The model under review builds one solid part; all positions refer to its coordinate system, in mm. Coordinates: 2 decimals unless noted, no trailing zeros. Order: outer loops, then holes, each group sorted by start corner. A loop starts at its lowest first (then second) coordinate and runs counter-clockwise, first axis right, second up.
from build123d import *

# Parameters (mm, degrees)
SKETCH1_W          = 127
SKETCH1_H          = 190.5
BASE_FLANGE1_DEPTH = 3.175
SKETCH7_R          = 2.54
SKETCH7_R_2        = 3.175
SKETCH7_R_3        = 14.2875
CUT_EXTRUDE1_DEPTH = 3.175
SKETCH10_R         = 2.54
CUT_EXTRUDE2_DEPTH = 115.52027386
CUT_EXTRUDE3_DEPTH = 115.52027386
CUT_EXTRUDE4_DEPTH = 115.52027386
SKETCH13_R         = 2.54
CUT_EXTRUDE5_DEPTH = 115.52027386


# Sheet-metal steps are written as plain solids
with BuildPart() as part:
    # Sketch1 → Base-Flange1 (new body)
    with BuildSketch(Plane(origin=(0, 0, 0), x_dir=(0, 0, -1), z_dir=(1, 0, 0))):
        Rectangle(SKETCH1_W, SKETCH1_H)
    extrude(amount=-BASE_FLANGE1_DEPTH)

    # Sketch7 → Cut-Extrude1 (cut)
    with BuildSketch(Plane(origin=(0, 0, 0), x_dir=(0, 0, -1), z_dir=(1, 0, 0))):
        with Locations((-28.380000009, -53.975)):
            Circle(SKETCH7_R)
        with Locations((28.380000009, -53.975)):
            Circle(SKETCH7_R)
        with Locations((0, 43.476657776)):
            Circle(SKETCH7_R_2)
        with Locations((0, -5.249171112)):
            Circle(SKETCH7_R_3)
    extrude(amount=-CUT_EXTRUDE1_DEPTH, mode=Mode.SUBTRACT)

    # Sketch10 → Cut-Extrude2 (cut, through all)
    with BuildSketch(Plane.ZY.offset(3.175)):
        with Locations((0, 34.740957442)):
            Circle(SKETCH10_R)
        with Locations((33.00000004, -3.749171064)):
            Circle(SKETCH10_R)
        with Locations((-33.00000004, -3.749171064)):
            Circle(SKETCH10_R)
        with Locations(Location((0, -45.239299666, 0), (0, 0, 180))):
            Circle(SKETCH10_R)
    extrude(amount=-CUT_EXTRUDE2_DEPTH, mode=Mode.SUBTRACT)

    # Sketch11 → Cut-Extrude3 (cut, through all)
    with BuildSketch(Plane.ZY.offset(3.175)):
        Polygon((-63.5, 95.25), (-63.5, -44.45), (19.05, 95.25), align=None)
    extrude(amount=-CUT_EXTRUDE3_DEPTH, mode=Mode.SUBTRACT)

    # Sketch12 → Cut-Extrude4 (cut, through all)
    with BuildSketch(Plane.ZY.offset(3.175)):
        Polygon((63.5, 50.8), (-7.215909091, 50.8), (19.05, 95.25), (63.5, 95.25), align=None)
    extrude(amount=-CUT_EXTRUDE4_DEPTH, mode=Mode.SUBTRACT)

    # Sketch13 → Cut-Extrude5 (cut, through all)
    with BuildSketch(Plane.ZY.offset(3.175)):
        with Locations((-50.8, -82.55)):
            Circle(SKETCH13_R)
        with Locations((0, -82.55)):
            Circle(SKETCH13_R)
        with Locations((50.8, -82.55)):
            Circle(SKETCH13_R)
        with Locations((-25.4, -82.55)):
            Circle(SKETCH13_R)
        with Locations((25.4, -82.55)):
            Circle(SKETCH13_R)
    extrude(amount=-CUT_EXTRUDE5_DEPTH, mode=Mode.SUBTRACT)


solid = part.part
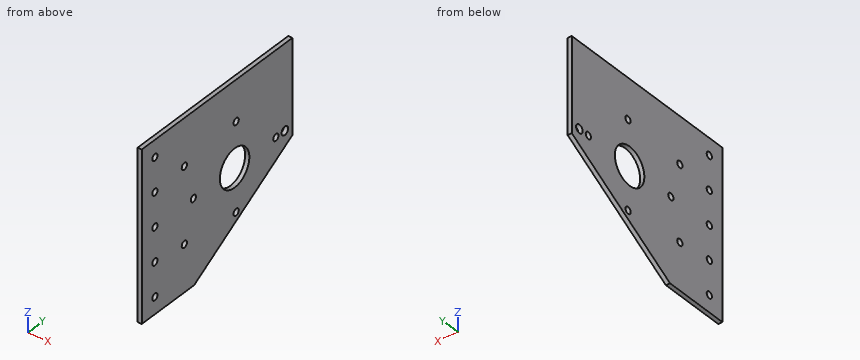
(1) Consider section C-C (z = -33). Give the boundary of the cut face in (x, y) (3 decimals), then the cut area to 3 significant figures.
(2) Consider section D-D (y = 23.5). Give the boundary of the cut face in (x, z) (3 decimals).
(3) Insertion check: pin 1 Ø6.5 at (y, z) = (-82.55, -50.8) entering from -X (3 decimals); pin 2 Ø1 at (x, y) = (-1, 30.5) entering from -Z. Each pin has a flat end and moves straight along its axis. Give the tip position at first contact, or say it passes through.
(4) Wall thickness on line 1 (Y direction, x = -1.05, z = 0); line 2 (Z direction, x = -0.85, y = -3); line 3 (Y direction, x = -2.7, z = -27.5): over which ranges is each line inside the solid? List them lowest first.
(5) Consider section B-B (x = -1.3). Give the number of separate pieces and of enclosed holes in the cut face, then the cut area to 3 significant figures.
(6) Consider section A-A (z = 33). Give the boundary of the cut face in (x, y) (3 decimals).
Findings:
1. outline: (-3.175, -95.25) - (0, -95.25) - (0, -6.289) - (-3.175, -6.289) - close; (-3.175, -1.209) - (0, -1.209) - (0, 7.165) - (-3.175, 7.165) - close
1. area: 309 mm2
2. outline: (-3.175, -23.348) - (0, -23.348) - (0, 63.5) - (-3.175, 63.5) - close
3. pin 1: stops at x = -3.175
3. pin 2: stops at z = -19.51
4. line 1: y = -95.25 to -85.09, -80.01 to -47.78, -42.7 to -19.54, 9.04 to 32.2, 37.28 to 40.3, 46.65 to 50.8
4. line 2: z = -39.01 to -35.43, -30.57 to -14.11, 14.11 to 30.57, 35.43 to 63.5
4. line 3: y = -95.25 to -83.98, -81.12 to -56.36, -51.59 to 16.47
5. separate pieces: 1
5. enclosed holes: 13
5. area: 15,000 mm2
6. outline: (-3.175, -95.25) - (0, -95.25) - (0, -6.289) - (-3.175, -6.289) - close; (-3.175, -1.209) - (0, -1.209) - (0, 50.8) - (-3.175, 50.8) - close
